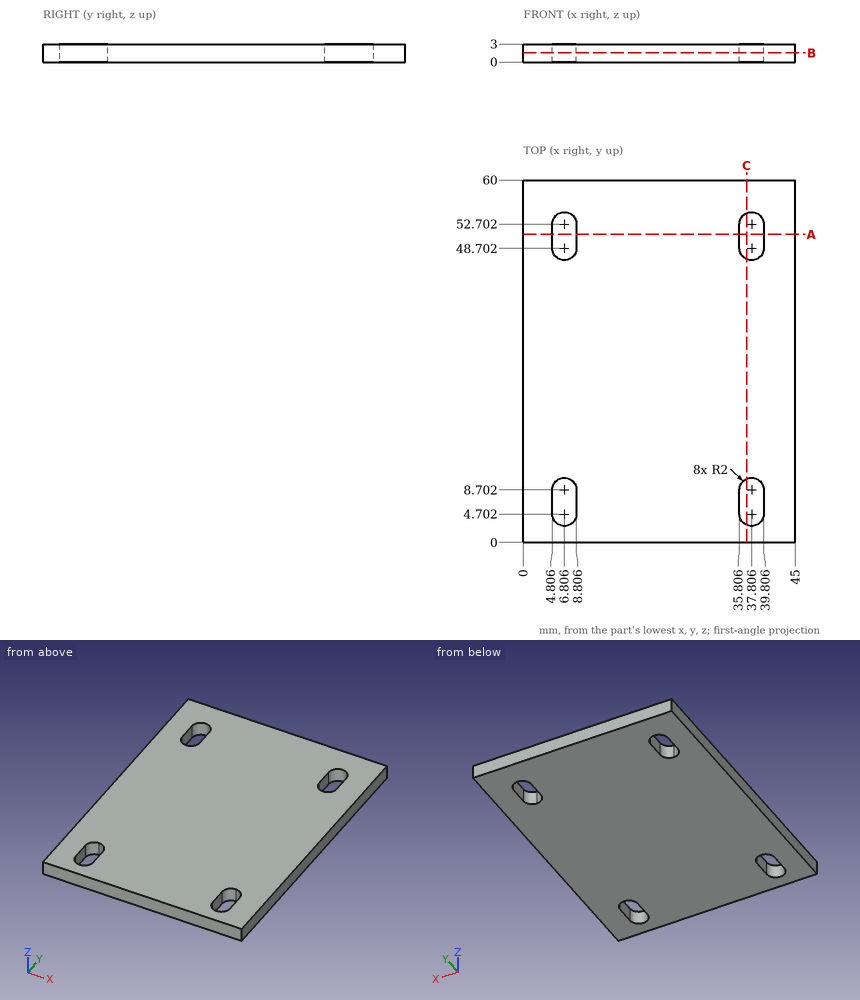
Can you work these out from the drawing? Everything is in mm from the part's minimum corner. Round coordinates to 2 decimals unless told otherwise and drop trailing zeros. Write each loop counter-clockwise with the first axis right and the second up, starting at its lowest first coordinate (ties: lowest second). Pieces come first, ordered by that corner, then holes. Notation, with made-up numbers: M -34.75,60 L 12.25,60 A15 cw 12.25,86 Z; hole C 4.25,-33 d9. An arc over 180 degrees is marked long. Use a Markdown table: item, result.
Item 1: If I drill on line 1 along X through (y, z) = (49, 1.75) (1 decimal); line 2 along Y through (x, z) = (38.5, 1.9) (1 decimal); line 3 along Y through (x, z) = (8.5, 2.3) (1 decimal), over which ranges is the centre line in solid material (lowest first)? Write a range as [from, to].
Found:
| item | result |
|---|---|
| line 1 | x = [0, 4.8], [8.8, 35.8], [39.8, 45] |
| line 2 | y = [0, 2.8], [10.6, 46.8], [54.6, 60] |
| line 3 | y = [0, 3.6], [9.8, 47.6], [53.8, 60] |
Item 2: I want a section at B-B (z = 1.55). List the corners of the cut face in (x, y) for me (1 decimal).
Found:
| item | result |
|---|---|
| outline | M 0,0 L 45,0 L 45,60 L 0,60 Z; hole M 4.8,4.7 A2 ccw 8.8,4.7 L 8.8,8.7 A2 ccw 4.8,8.7 Z; hole M 4.8,48.7 A2 ccw 8.8,48.7 L 8.8,52.7 A2 ccw 4.8,52.7 Z; hole M 35.8,4.7 A2 ccw 39.8,4.7 L 39.8,8.7 A2 ccw 35.8,8.7 Z; hole M 35.8,48.7 A2 ccw 39.8,48.7 L 39.8,52.7 A2 ccw 35.8,52.7 Z |
Item 3: I want a section at A-A (y = 51). List the corners of the cut face in (x, z) for me (1 decimal).
Found:
| item | result |
|---|---|
| outline | M 0,0 L 4.8,0 L 4.8,3 L 0,3 Z; M 8.8,0 L 35.8,0 L 35.8,3 L 8.8,3 Z; M 39.8,0 L 45,0 L 45,3 L 39.8,3 Z |
Item 4: I want a section at C-C (x = 37). List the corners of the cut face in (y, z) for me, and give its area (3 significant figures).
Found:
| item | result |
|---|---|
| outline | M 0,0 L 2.87,0 L 2.87,3 L 0,3 Z; M 10.53,0 L 46.87,0 L 46.87,3 L 10.53,3 Z; M 54.53,0 L 60,0 L 60,3 L 54.53,3 Z |
| area | 134 mm2 |
